Part model, mm, in its own coordinate system. Face numbers are marked on the shaded views. A direction names the side the tool comes from. Give positions to 0.01 mm unless a question says otherwise; leave off trailing zeros. Write each loop counter-clockwise with the first axis right and the second up, starting at its lowest first coordinate (ties: lowest second). Pieces come first, ordered by that corner, then holes. Notation, with made-up numbers: (2, 0) - (28, 0) arc R34 cw to (28, 38) - close; hole circle Ø9 at (12.5, -38.75). An arc over 180 degrees is marked (long way). Answer as a JSON object with one key per item and string values. Group by question number.
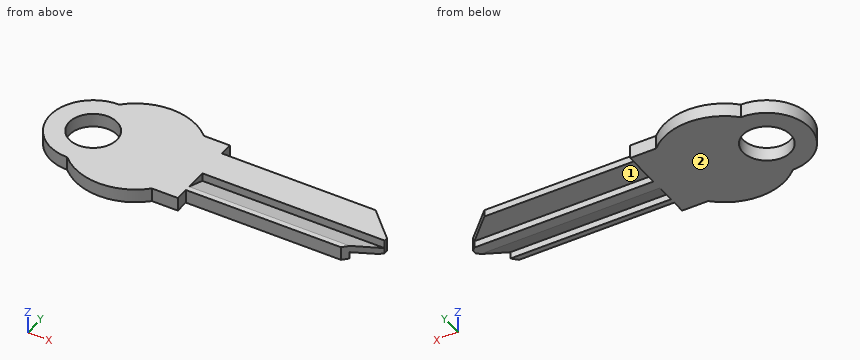
```python
from build123d import *

# Parameters (mm, degrees)
F0_R     = 3.5
F1_DEPTH = 2
F3_DEPTH = 26.7
F5_DEPTH = 2.001


with BuildPart() as f1:
    # F0 (on Top) → F1 (new body)
    with BuildSketch(Plane.XY):
        with BuildLine():
            Line((6.2, -6.3), (10, -6.3))
            Line((10, -6.3), (10, 6.3))
            Line((10, 6.3), (6.2, 6.3))
            ThreePointArc((6.2, 6.3), (0, 8.839118), (-6.2, 6.3))
            ThreePointArc((-6.2, 6.3), (-12.5, 0), (-6.2, -6.3))
            ThreePointArc((-6.2, -6.3), (0, -8.839118), (6.2, -6.3))
        make_face()
        with Locations((-6.2, 0)):
            Circle(F0_R, mode=Mode.SUBTRACT)
    extrude(amount=F1_DEPTH)

    # F2 (on face) → F3 (join)
    with BuildSketch(Plane.YZ.offset(10)):
        Polygon((-0.875, 0), (0.675, 0), (0.675, 1), (4.375, 1), (4.375, 2), (-0.375, 2), (-0.375, 0.8), (-3.575, 2), (-4.375, 2), (-4.375, 0), (-3.575, 0), (-3.575, 1), align=None)
    extrude(amount=F3_DEPTH)

    # F4 (on face) → F5 (cut, through all)
    with BuildSketch(Plane.XY.offset(2)):
        Polygon((36.7, 0.175), (36.7, 4.375), (32.5, 4.375), align=None)
        Polygon((32.7, -4.375), (36.7, -4.375), (36.7, -0.375), align=None)
    extrude(amount=-F5_DEPTH, mode=Mode.SUBTRACT)


solid = f1.part
```
1) Drop flat-ended pins along their axis: P1, Ø0.8, axis at x = 19, z = 0.5, coming from the +Y side (3 decimals); P2, Ø0.8, axis at x = 25, z = 1.5, coming from the +Y side (3 decimals); P3, Ø0.6, axis at y = 2.5, z = 1.5, coming from the +X side (3 decimals); P4, Ø5.5, axis at x = -6.2, y = 0, coming from the +Z side. Give the stop position or say it passes through.
2) Probe line 1 (X direction, y = -2.25, z = 0.65) (3 decimals); line 2 (Y direction, x = -5, z = 1.75); line 3 (X direction, y = 0.5, z = 0.1) (3 decimals). List the from-to ranges inside material, lowest first.
3) Band-saw the part on A-A (x = 29). List the corners of the cut face in (y, z) (3 decimals), plus the area to 3 significant figures.
4) Band-saw the part on B-B (z = 1.7). List the corners of the cut face in (x, y) (3 decimals).
5) Which spindle directions (+Z, -Z, +X, -X, +Y, -Y) get a long thin tool onto all of the face, cutting with end or side? Do the marked faces 1 and 2. Say none if no direction does.
6) Band-saw the part on D-D (y = -5.25). List the corners of the cut face in (x, z).
7) Band-saw the part on C-C (y = 3). List the corners of the cut face in (x, z) (3 decimals).
Verdict:
{
 "1": {"P1": "y = 0.675", "P2": "y = 4.375", "P3": "x = 34.675", "P4": "through"},
 "2": {"line 1": "-12.085 to -8.881, -3.519 to 34.825", "line 2": "-7.29 to -3.29, 3.29 to 7.29", "line 3": "-12.48 to -9.664, -2.736 to 36.375"},
 "3": {"outline": "(-4.375, 0) - (-3.575, 0) - (-3.575, 1) - (-0.875, 0) - (0.675, 0) - (0.675, 1) - (4.375, 1) - (4.375, 2) - (-0.375, 2) - (-0.375, 0.8) - (-3.575, 2) - (-4.375, 2) - close", "area": "10.5 mm2"},
 "4": {"outline": "(-6.2, -6.3) arc R8.839 ccw to (6.2, -6.3) - (10, -6.3) - (10, -4.375) - (32.7, -4.375) - (34.3, -2.775) - (10, -2.775) - (10, -0.375) - (36.7, -0.375) - (36.7, 0.175) - (32.5, 4.375) - (10, 4.375) - (10, 6.3) - (6.2, 6.3) arc R8.839 ccw to (-6.2, 6.3) arc R6.3 ccw to start; hole circle Ø7 at (-6.2, 0)"},
 "5": {"face 1": "-Z, +X, +Y", "face 2": "-Z, +X, -X, +Y, -Y"},
 "6": {"outline": "(-9.68, 0) - (10, 0) - (10, 2) - (-9.68, 2) - close"},
 "7": {"outline": "(-11.74, 0) - (-8.003, 0) - (-8.003, 2) - (-11.74, 2) - close; (-4.397, 0) - (10, 0) - (10, 1) - (33.875, 1) - (33.875, 2) - (-4.397, 2) - close"}
}
